Verification items for the finished model (mm, model axes). A direction names the side the tool comes from. Round coordinates to 2 decimals unless told otherwise and drop trailing zeros. Loops run counter-clockwise (first coordinate to the right, second up) from the corner with the lowest first, then second, coordinate; pieces in that order, holes last. Notation, with made-up numbers: M -14.75,28.5 L 30.25,28.5 A17 cw 30.25,51.5 Z; hole C 77,50.5 d4. An arc over 180 degrees is marked long. One line per item, written item: value.
from build123d import *

# Parameters (mm, degrees)
F1_DEPTH = 15
F2_W     = 10
F2_H     = 10.395046
F2_H_2   = 10.143298
F3_DEPTH = 40
F4_W     = 3.51127
F4_H     = 10
F5_DEPTH = 10.143298
F6_R     = 3.75
F7_DEPTH = 25


with BuildPart() as f1:
    # F0 (on Front) → F1 (new body)
    with BuildSketch(Plane.XZ):
        Polygon((0, 12.643298), (0, 0), (36.2, 0), (28.900388, 12.643298), (18.709274, 18.527141), (9.287707, 18.527141), (9.287707, 12.643298), align=None)
    extrude(amount=F1_DEPTH)

    # F2 (on face) → F3 (cut)
    with BuildSketch(Plane(origin=(0, 0, 0), x_dir=(0, -1, 0), z_dir=(-1, 0, 0))):
        with Locations((7.5, 17.840821)):
            Rectangle(F2_W, F2_H)
        with Locations((7.5, 7.571649)):
            Rectangle(F2_W, F2_H_2)
    extrude(amount=-F3_DEPTH, mode=Mode.SUBTRACT)

    # F4 (on face) → F5 (join, through all)
    with BuildSketch(Plane.XY.offset(2.5)):
        with Locations((1.755635, -7.5)):
            Rectangle(F4_W, F4_H)
    extrude(amount=F5_DEPTH)

    # F6 (on face) → F7 (cut)
    with BuildSketch(Plane.XZ.offset(15)):
        with Locations((15.891228, 8.597537)):
            Circle(F6_R)
    extrude(amount=-F7_DEPTH, mode=Mode.SUBTRACT)


solid = f1.part
(1) Tool access check on faces 1 (the face through (12.145, -1.268, 8.762)), 2 (the face through (9.288, -1, 16)), 3 (the face through (19, -7, 2.5)). Record the directions out of +Z, -Z, +X, -X, +Y, -Y that give a thin tool (end or side, any length) a straight path to the whole face; none if there is none.
Completed:
face 1: +Y, -Y
face 2: +Z, -X, +Y, -Y
face 3: +Z, +X
(2) Sectioned sample at C-C on x = 7.5. Enter the section's corners in (y, z), and give its area (3 significant figures).
Completed:
outline: M -15,0 L 0,0 L 0,12.64 L -2.5,12.64 L -2.5,2.5 L -12.5,2.5 L -12.5,12.64 L -15,12.64 Z
area: 88.2 mm^2
(3) Thickness scan on L1, parallel to Y at x = 21, z = 15.5; L2, parallel to Z at x = 26, y = -3; L3, parallel to X at y = -10.5, z = 6.5. Record the ranges inside material, lowest first. Write a range as from..to.
Completed:
L1: y = -15..-12.5, -2.5..0
L2: z = 0..2.5
L3: x = 0..3.51
(4) Mould release check, pull along Y, two halves, no side actions. Record for faces 4 (the face through (18, -15, 5)), 5 (the face through (18, 0, 5)), 6 (the face through (14, -14, 18.527)), 7 (the face through (3.511, -8, 8)): +Y half, -Y half, draft (parallel to the pull), parting line (faces both ways), or undercut.
Completed:
face 4: -Y half
face 5: +Y half
face 6: draft
face 7: undercut
(5) Sectioned sample at D-D on y = -8.5. Enter the section's corners in (x, z), and give its area (3 significant figures).
Completed:
outline: M 0,0 L 36.2,0 L 34.76,2.5 L 3.51,2.5 L 3.51,12.64 L 0,12.64 Z
area: 124 mm^2
(6) Sectioned sample at B-B on x = 16. Enter the section's corners in (y, z), and give its area (3 significant figures).
Completed:
outline: M -15,0 L 0,0 L 0,4.85 L -2.5,4.85 L -2.5,2.5 L -12.5,2.5 L -12.5,4.85 L -15,4.85 Z; M -15,12.35 L -12.5,12.35 L -12.5,18.53 L -15,18.53 Z; M -2.5,12.35 L 0,12.35 L 0,18.53 L -2.5,18.53 Z
area: 80.2 mm^2
(7) Sectioned sample at A-A on z = 15.75. Enter the section's corners in (x, y), and give its area (3 significant figures).
Completed:
outline: M 9.29,-15 L 23.52,-15 L 23.52,-12.5 L 9.29,-12.5 Z; M 9.29,-2.5 L 23.52,-2.5 L 23.52,0 L 9.29,0 Z
area: 71.2 mm^2
(8) Depth check by flat-ended pin: pin 1 Ø5 at (x, y) = (17.5, -7) entering from +Z; pin 2 Ø4.5 at (x, y) = (4.5, -6.5) entering from +Z; pin 3 Ø1.2 at (y, z) = (-13.5, 14.5) entering from -X; pin 4 Ø4.5 at (x, z) = (15.89, 8.6) entering from -Y. Enter the tip coordinate at first touch or a pass-through.
Completed:
pin 1: stops at z = 2.5
pin 2: stops at z = 12.64
pin 3: stops at x = 9.29
pin 4: passes through
